Design review of the part built by this model. Coordinates are the model's own, in mm. Coordinates: 2 decimals unless noted, no trailing zeros. Write each loop counter-clockwise with the first axis right and the second up, starting at its lowest first coordinate (ties: lowest second). Pieces come first, ordered by that corner, then holes. Notation, with made-up numbers: (79, 21.25) - (89, 21.25) arc R21 cw to (89, 38.25) - close; hole circle Ø9 at (70.25, 13). An arc over 180 degrees is marked (long way). One line per item, written item: value.
from build123d import *

# Parameters (mm, degrees)
F0_W     = 25.4
F0_H     = 19.05
F0_R     = 2.7432
F1_DEPTH = 4.7625
F2_SIZE  = 1.524


with BuildPart() as f1:
    # F0 (on Top) → F1 (new body)
    with BuildSketch(Plane.XY):
        Rectangle(F0_W, F0_H)
        with Locations((-6.35, 0)):
            Circle(F0_R, mode=Mode.SUBTRACT)
        with Locations((6.35, 0)):
            Circle(F0_R, mode=Mode.SUBTRACT)
    extrude(amount=F1_DEPTH)

    # F2
    f2_edges = [f1.edges().sort_by_distance(p)[0] for p in [
        (-9.0932, 0, 4.7625),
        (3.6068, 0, 4.7625),
    ]]
    chamfer(f2_edges, length=F2_SIZE)


solid = f1.part
1. Mouldability with a two-part tool opening along X and no side actions: class faces 1 (the face through (-3.733, 0.824, 1.597)), 2 (the face through (-12.7, 0, 2)), 3 (the face through (0, 0, 0)) as released by +X, released by -X, zero draft, split by the parting line, or undercut.
Answer block:
face 1: undercut
face 2: released by -X
face 3: zero draft
2. Consider section B-B, the plane z = 1.75. Write out the cut boundary in (x, y) (3 decimals), then the cut area to 3 significant figures.
Answer block:
outline: (-12.7, -9.525) - (12.7, -9.525) - (12.7, 9.525) - (-12.7, 9.525) - close; hole circle Ø5.486 at (-6.35, 0); hole circle Ø5.486 at (6.35, 0)
area: 437 mm^2
3. Consider section D-D, the plane z = 4.3. Write out the cut boundary in (x, y) (3 decimals).
Answer block:
outline: (-12.7, -9.525) - (12.7, -9.525) - (12.7, 9.525) - (-12.7, 9.525) - close; hole circle Ø7.609 at (-6.35, 0); hole circle Ø7.609 at (6.35, 0)
4. Consider section C-C, the plane x = 6.35. Write out the cut boundary in (y, z) (1 decimal).
Answer block:
outline: (-9.5, 0) - (-2.7, 0) - (-2.7, 3.2) - (-4.3, 4.8) - (-9.5, 4.8) - close; (2.7, 0) - (9.5, 0) - (9.5, 4.8) - (4.3, 4.8) - (2.7, 3.2) - close
5. Wall thickness on line 1 along Y through (x, z) = (6.35, 0.75) (3 decimals); line 2 along X through (y, z) = (2, 0.9); line 3 along X through (y, z) = (2.5, 2.9): over which ranges is each line inside the solid? List them lowest first.
Answer block:
line 1: y = -9.525 to -2.743, 2.743 to 9.525
line 2: x = -12.7 to -8.23, -4.47 to 4.47, 8.23 to 12.7
line 3: x = -12.7 to -7.48, -5.22 to 5.22, 7.48 to 12.7
6. Consider section A-A, the plane y = 0. Write out the cut boundary in (x, z), then the cut area to 3 significant figures.
Answer block:
outline: (-12.7, 0) - (-9.09, 0) - (-9.09, 3.24) - (-10.62, 4.76) - (-12.7, 4.76) - close; (-3.61, 0) - (3.61, 0) - (3.61, 3.24) - (2.08, 4.76) - (-2.08, 4.76) - (-3.61, 3.24) - close; (9.09, 0) - (12.7, 0) - (12.7, 4.76) - (10.62, 4.76) - (9.09, 3.24) - close
area: 64.1 mm^2
7. Insertion check: pin 1 Ø5 at (x, y) = (2.5, 1.5) entering from -Z. The pin has a flat end and moves straight along its axis. Give the tip position at first contact, or say it passes through.
Answer block:
pin 1: stops at z = 0
